Drawing for the job (mm, zero at the part's lowest x, y, z). A direction names the side the tool comes from. Round coordinates to 2 decimals unless told otherwise and drop trailing zeros. Loops run counter-clockwise (first coordinate to the right, second up) from the corner with the lowest first, then second, coordinate; pieces in that order, holes last. Notation, with made-up numbers: M -12,86 L 43,86 A26 ccw 43,103 Z; hole C -37,35.5 d1. An arc over 180 degrees is marked long. Answer in a Markdown table with one row per item.
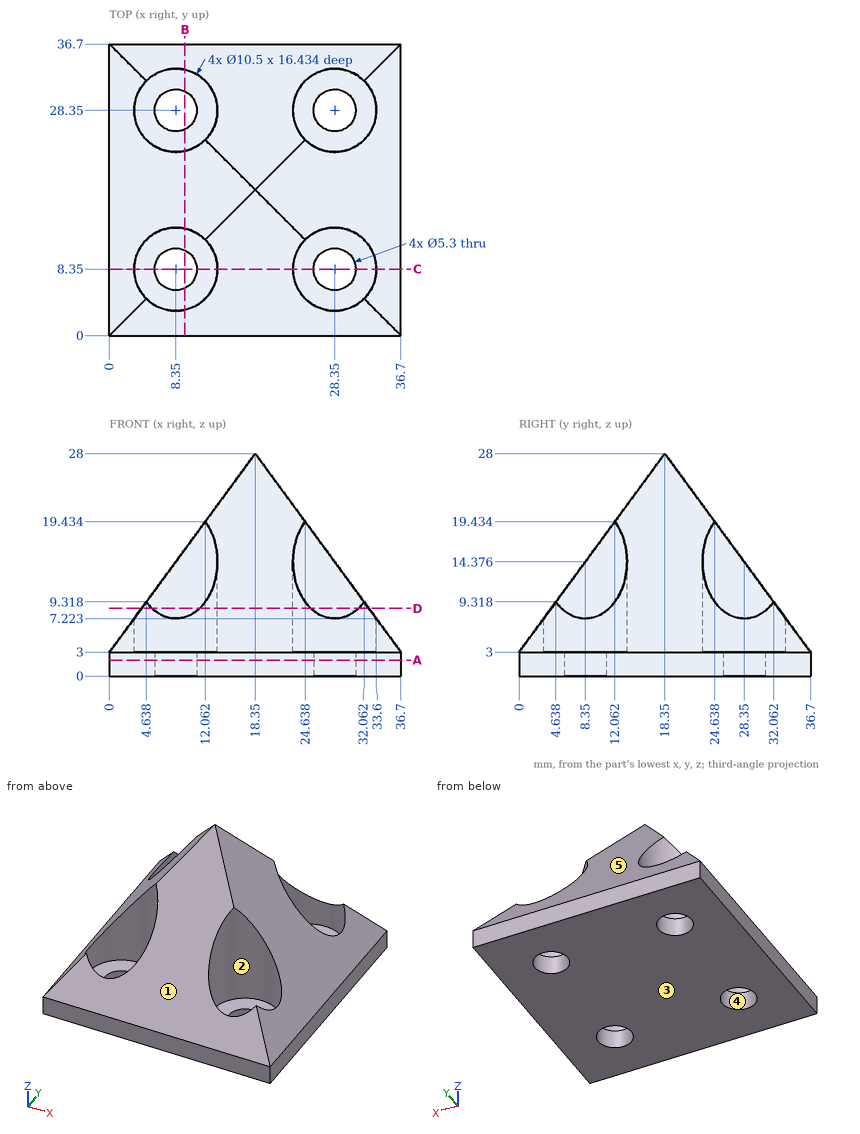
1. Pin check, flat tips, straight feed: pin 1 (8.5 mm diameter, centred on x = 28.35, y = 28.35, fed in from +Z); pin 2 (1 mm diameter, centred on y = 6.5, z = 7, fed in from -X); pin 3 (10 mm diameter, centred on y = 17, z = 13.5, fed in from +X); pin 4 (5 mm diameter, centred on x = 8.35, y = 8.35, fed in from +Z). Stop position of each tip, or through.
Verdict:
| item | result |
|---|---|
| pin 1 | stops at z = 3 |
| pin 2 | stops at x = 2.57 |
| pin 3 | stops at x = 32.66 |
| pin 4 | passes through |
2. Saw through at A-A (z = 2). Write the cut outline in (x, y).
Verdict:
| item | result |
|---|---|
| outline | M 0,0 L 36.7,0 L 36.7,36.7 L 0,36.7 Z; hole C 8.35,8.35 d5.3; hole C 8.35,28.35 d5.3; hole C 28.35,8.35 d5.3; hole C 28.35,28.35 d5.3 |
3. Wall check: probe 1 along Y at (x, z) = (28.35, 0.9); probe 2 along Y at (x, z) = (28.35, 6.5); probe 3 along Y at (x, z) = (28.35, 9.25). Give the ranges that are in metal, low to high.
Verdict:
| item | result |
|---|---|
| probe 1 | y = 0 to 5.7, 11 to 25.7, 31 to 36.7 |
| probe 2 | y = 2.57 to 3.1, 13.6 to 23.1, 33.6 to 34.13 |
| probe 3 | y = 13.6 to 23.1 |
4. Saw through at C-C (y = 8.35). Write the cut outline in (x, z).
Verdict:
| item | result |
|---|---|
| outline | M 0,0 L 5.7,0 L 5.7,3 L 3.1,3 L 3.1,7.22 L 0,3 Z; M 11,0 L 25.7,0 L 25.7,3 L 23.1,3 L 23.1,14.38 L 13.6,14.38 L 13.6,3 L 11,3 Z; M 31,0 L 36.7,0 L 36.7,3 L 33.6,7.22 L 33.6,3 L 31,3 Z |
5. Saw through at B-B (x = 9.5). Write the cut outline in (y, z), and give its area (3 significant figures).
Verdict:
| item | result |
|---|---|
| outline | M 0,0 L 5.96,0 L 5.96,3 L 3.23,3 L 3.23,7.4 L 0,3 Z; M 10.74,0 L 25.96,0 L 25.96,3 L 23.23,3 L 23.23,15.94 L 13.47,15.94 L 13.47,3 L 10.74,3 Z; M 30.74,0 L 36.7,0 L 36.7,3 L 33.47,7.4 L 33.47,3 L 30.74,3 Z |
| area | 222 mm² |
6. Mould opens along Y. For the marked faces 3, 4 and 5 say: +Y half, -Y half, draft (parallel to the pull), parting line (faces both ways), or undercut.
Verdict:
| item | result |
|---|---|
| face 3 | draft |
| face 4 | undercut |
| face 5 | +Y half |
7. Saw through at D-D (z = 8.5). Write the cut outline in (x, y).
Verdict:
| item | result |
|---|---|
| outline | M 4.04,4.04 L 5.36,4.04 A5.25 cw 4.04,5.36 Z; M 4.04,11.34 A5.25 cw long 11.34,4.04 L 25.36,4.04 A5.25 cw long 32.66,11.34 L 32.66,25.36 A5.25 cw long 25.36,32.66 L 11.34,32.66 A5.25 cw long 4.04,25.36 Z; M 4.04,31.34 A5.25 cw 5.36,32.66 L 4.04,32.66 Z; M 31.34,4.04 L 32.66,4.04 L 32.66,5.36 A5.25 cw Z; M 31.34,32.66 A5.25 cw 32.66,31.34 L 32.66,32.66 Z |
8. Tool access for the marked faces 1 and 2: list every direction of +Z, -Z, +X, -X, +Y, -Y with a clear straight run to the whole face (end or side of a thin tool).
Verdict:
| item | result |
|---|---|
| face 1 | +Z, +X, -X, -Y |
| face 2 | +Z |
